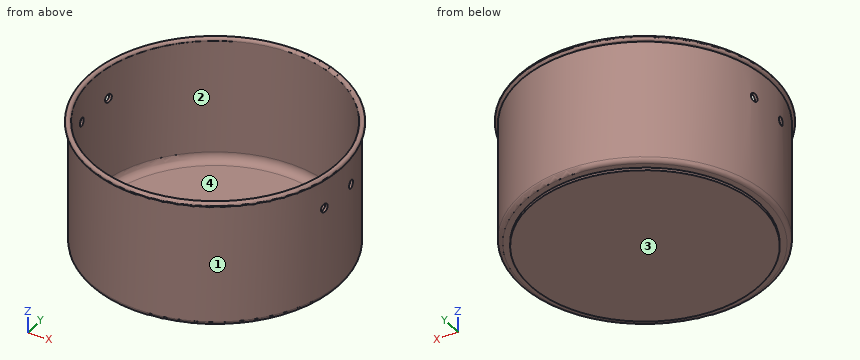
```python
from build123d import *

# Parameters (mm, degrees)
F0_W     = 69.85
F0_H     = 1.5875
F2_R     = 5.08
F3_R     = 2.54
F5_R     = 2.54
F6_DEPTH = 228.854
F7_DEPTH = 243.84


with BuildPart() as f1:
    # F0 (on Front) → F1 (revolve)
    with BuildSketch(Plane.XZ):
        with BuildLine():
            Line((0, 1.5875), (0, 0))
            Line((0, 0), (69.85, 0))
            Line((69.85, 0), (76.2, 0))
            Line((76.2, 0), (76.2, 74.6125))
            ThreePointArc((76.2, 74.6125), (75.077468, 75.077468), (74.6125, 76.2))
            Line((74.6125, 76.2), (74.6125, 1.5875))
            Line((74.6125, 1.5875), (0, 1.5875))
        make_face()
        with Locations((34.925, -0.79375)):
            Rectangle(F0_W, F0_H)
        with BuildLine():
            ThreePointArc((74.6125, 76.2), (75.077468, 75.077468), (76.2, 74.6125))
            ThreePointArc((76.2, 74.6125), (77.322532, 75.077468), (77.7875, 76.2))
            ThreePointArc((77.7875, 76.2), (76.2, 77.7875), (74.6125, 76.2))
        make_face()
    revolve(axis=Axis((0, 0, 12.051039), (0, 0, 1)))

    # F2
    f2_edges = [f1.edges().sort_by_distance(p)[0] for p in [
        (-74.6125, 0, 1.5875),
    ]]
    fillet(f2_edges, radius=F2_R)

    # F3
    f3_edges = [f1.edges().sort_by_distance(p)[0] for p in [
        (-76.2, 0, 0),
    ]]
    fillet(f3_edges, radius=F3_R)

    # F5 (on offset) → F6 (cut)
    with BuildSketch(Plane.YZ.offset(101.6)):
        with Locations((-12.954, 56.800925)):
            Circle(F5_R)
    extrude(amount=-F6_DEPTH, mode=Mode.SUBTRACT)

    # F5 (on offset) → F7 (cut)
    with BuildSketch(Plane.YZ.offset(101.6)):
        with Locations((12.954, 56.800925)):
            Circle(F5_R)
    extrude(amount=-F7_DEPTH, mode=Mode.SUBTRACT)


solid = f1.part
```
Model file for the job. Use its own axes, mm. Face numbers are marked on the shaded views. Give positions to 0.01 mm unless a question says otherwise; leave off trailing zeros. Order: outer loops, then holes, each group sorted by start corner. A loop starts at its lowest first (then second) coordinate and runs counter-clockwise, first axis right, second up.
1) Mould opens along X. For the marked faces 1, 2, 3 and 4 say: +X half, -X half, draft (parallel to the pull), parting line (faces both ways), or undercut.
2) Saw through at A-A, the plane z = 51. Write the cut outline in (x, y) (1 decimal).
3) Pin check, flat tips, straight feed: pin 1 (2 mm diameter, centred on x = 9.5, y = 52.5, fed in from +Z); pin 2 (8 mm diameter, centred on y = 12.95, z = 56.8, fed in from +X); pin 3 (6 mm diameter, centred on y = 12.95, z = 56.8, fed in from -X); pin 4 (3 mm diameter, centred on y = -12.95, z = 56.8, fed in from -X). Stop position of each tip, or through.
4) Saw through at B-B, the plane y = -13.5. Count the separate pieces of the cut face and the enclosed holes in it, then the cut area to 3 significant figures.
5) Wall check: probe 1 along Y at (x, z) = (0, 55); probe 2 along X at (y, z) = (56, 57); probe 3 along Z at (x, y) = (12, -14). Give the ranges that are in metal, low to high.
Computed:
1. face 1: parting line
1. face 2: undercut
1. face 3: draft
1. face 4: undercut
2. outline: circle Ø152.4 at (0, 0); hole circle Ø149.2 at (0, 0)
3. pin 1: stops at z = 1.59
3. pin 2: stops at x = 75.67
3. pin 3: stops at x = -75.55
3. pin 4: passes through
4. separate pieces: 3
4. enclosed holes: 0
4. area: 701 mm2
5. probe 1: y = -76.2 to -74.61, 74.61 to 76.2
5. probe 2: x = -51.68 to -49.31, 49.31 to 51.68
5. probe 3: z = -1.59 to 1.59
